```python
from build123d import *

# Parameters (mm, degrees)
F0_W      = 52
F0_H      = 41
F1_DEPTH  = 4
F2_W      = 5.1310285926
F2_H      = 4.6637309715
F3_DEPTH  = 34
F4_DEPTH  = 18
F5_W      = 4.6637309715
F5_H      = 4.0902358592
F6_DEPTH  = 21.88
F7_W      = 4.6637309715
F7_H      = 3.8742293864
F8_DEPTH  = 21.88
F10_DEPTH = 4.5


with BuildPart() as f1:
    # F0 (on Top) → F1 (new body)
    with BuildSketch(Plane.XY):
        with Locations((-25.150391832, 1.4550268714)):
            Rectangle(F0_W, F0_H)
    extrude(amount=F1_DEPTH)

    # F2 (on face) → F3 (join)
    with BuildSketch(Plane.XY.offset(4)):
        with Locations((-26.7044808716, 18.0663228966)):
            Rectangle(F2_W, F2_H)
    extrude(amount=F3_DEPTH)

    # F2 (on face) → F4 (join)
    with BuildSketch(Plane.XY.offset(4)):
        with Locations((-26.7044808716, -15.3699782677)):
            Rectangle(F2_W, F2_H)
    extrude(amount=F4_DEPTH)

    # F5 (on face) → F6 (join)
    with BuildSketch(Plane(origin=(-29.2699951679, 0, 0), x_dir=(0, -1, 0), z_dir=(-1, 0, 0))):
        with Locations((-18.0663228966, 35.9548820704)):
            Rectangle(F5_W, F5_H)
    extrude(amount=F6_DEPTH)

    # F7 (on face) → F8 (join)
    with BuildSketch(Plane(origin=(-29.2699951679, 0, 0), x_dir=(0, -1, 0), z_dir=(-1, 0, 0))):
        with Locations((15.3699782677, 20.0628853068)):
            Rectangle(F7_W, F7_H)
    extrude(amount=F8_DEPTH)

    # F9 (on face) → F10 (join)
    with BuildSketch(Plane(origin=(-51.1499951679, 0, 0), x_dir=(0, -1, 0), z_dir=(-1, 0, 0))):
        Polygon((14.0116587281, 21.4774478227), (-15.7344574109, 38), (-15.7344574109, 33.9097641408), (13.0349043757, 18.1450489908), (14.0116587281, 18.1450489908), align=None)
    extrude(amount=-F10_DEPTH)

    # F11: F1 across face


with BuildPart() as f1_1:
    add(f1.part)
    add(f1.part.mirror(Plane(origin=(0.849608168, 1.4550268714, 2), x_dir=(0, 1, 0), z_dir=(1, 0, 0))))


solid = f1_1.part
```
Input: part model. Units: mm. Frame: model coordinates. A direction names the side the tool comes from. Give positions to 0.01 mm unless a question says otherwise; leave off trailing zeros. Order: outer loops, then holes, each group sorted by start corner. A loop starts at its lowest first (then second) coordinate and runs counter-clockwise, first axis right, second up. Notation, with made-up numbers: M 26.25,18 L 82.25,18 A24 cw 82.25,49 Z; hole C 77,51.25 d6. An arc over 180 degrees is marked long. One line per question, with ' | ' between items. Start each with the question number.
1. Access query for faces 1 (the face through (-40, -15, 18.126)), 2 (the face through (42, 18, 33.91)), 3 (the face through (-40, 18, 33.91)), 4 (the face through (25.838, 18, 21)), 5 (the face through (30.969, -15, 11)). Directions: +Z, -Z, +X, -X, +Y, -Y. A direction counts if a zero-diameter tool reaches every point of the face in a straight line with its end or side. Return the directions, or none.
2. Material intervals for probe 1 along X at (y, z) = (6.5, 30); probe 2 along Z at (x, y) = (-47, 17); probe 3 along X at (y, z) = (17.5, 5.5), sorted ascending. Write a range as [from, to].
3. Section query C-C (x = 40). Return the cut outline in (y, z).
4. Section query D-D (z = 20). Return the cut outline in (x, y), and give its area (3 significant figures).
5. First-contact query: pin 1 Ø10 at (x, y) = (-37, -8.5) entering from +Z; pin 2 Ø6 at (y, z) = (17, 10.5) entering from -X; pin 3 Ø1.4 at (y, z) = (17, 24) entering from +X. Flat tips, straight axial feed; report the tip coordinate or a pass-through.
6. Pull-direction query (Y, two-part tool) for faces 6 (the face through (30, 20.398, 26)), 7 (the face through (30, 15.734, 23)), 8 (the face through (-37, 18, 38)), 9 (the face through (2, -19.045, 2)); classes: released by +Y, released by -Y, zero draft, split by the parting line, or undercut.
7. Section query A-A (y = 10.5). Return the cut outline in (x, z).
8. Section query B-B (z = 11.5). Return the cut outline in (x, y).
Here are the results:
1) face 1: -X, +Y, -Y | face 2: +X, +Y | face 3: -X, +Y | face 4: +Z, +Y, -Y | face 5: +X, +Y, -Y
2) probe 1: [-51.15, -46.65], [48.35, 52.85] | probe 2: [0, 4], [33.91, 38] | probe 3: [-29.27, -24.14], [25.84, 30.97]
3) outline: M -19.04,0 L 21.96,0 L 21.96,4 L -19.04,4 Z; M -17.7,18.13 L -13.04,18.13 L -13.04,22 L -17.7,22 Z; M 15.73,33.91 L 20.4,33.91 L 20.4,38 L 15.73,38 Z
4) outline: M -51.15,-17.7 L -24.14,-17.7 L -24.14,-13.04 L -46.65,-13.04 L -46.65,-9.65 L -51.15,-9.65 Z; M -29.27,15.73 L -24.14,15.73 L -24.14,20.4 L -29.27,20.4 Z; M 25.84,-17.7 L 52.85,-17.7 L 52.85,-9.65 L 48.35,-9.65 L 48.35,-13.04 L 25.84,-13.04 Z; M 25.84,15.73 L 30.97,15.73 L 30.97,20.4 L 25.84,20.4 Z | area: 330 mm²
5) pin 1: z = 22 | pin 2: x = -29.27 | pin 3: x = 30.97
6) face 6: released by +Y | face 7: undercut | face 8: zero draft | face 9: released by -Y
7) outline: M -51.15,0 L 52.85,0 L 52.85,4 L -51.15,4 Z; M -51.15,31.04 L -46.65,31.04 L -46.65,35.09 L -51.15,35.09 Z; M 48.35,31.04 L 52.85,31.04 L 52.85,35.09 L 48.35,35.09 Z
8) outline: M -29.27,-17.7 L -24.14,-17.7 L -24.14,-13.04 L -29.27,-13.04 Z; M -29.27,15.73 L -24.14,15.73 L -24.14,20.4 L -29.27,20.4 Z; M 25.84,-17.7 L 30.97,-17.7 L 30.97,-13.04 L 25.84,-13.04 Z; M 25.84,15.73 L 30.97,15.73 L 30.97,20.4 L 25.84,20.4 Z
